Geometry: final body of the model. Coordinates: model frame, mm. A direction names the side the tool comes from. Give positions to 0.01 mm unless a question says otherwise; leave off trailing zeros. Write each loop counter-clockwise with the first axis right and the second up, starting at its lowest first coordinate (ties: lowest second). Pieces come first, ordered by that corner, then holes. Notation, with made-up numbers: (81.25, 5.25) -> (98.25, 5.25) arc R27 ccw to (98.25, 39.25) -> close; hole circle Ø11 at (-36, 45.25). An arc over 180 degrees is marked (long way). Answer in a Markdown table with one row per item. Add a question column.
from build123d import *

# Parameters (mm, degrees)
F1_DEPTH = 63.5
F2_DEPTH = 7.9375
F0_W     = 25.4
F0_H     = 19.05
F3_DEPTH = 25.4


with BuildPart() as f1:
    # F0 (on Front) → F1 (new body, symmetric)
    with BuildSketch(Plane.XZ):
        Polygon((22.225, 9.525), (-41.275, 9.525), (-41.275, -9.525), (41.275, -9.525), (41.275, 9.525), align=None)
    extrude(amount=F1_DEPTH, both=True)

    # F0 (on Front) → F2 (join, symmetric)
    with BuildSketch(Plane.XZ):
        with BuildLine():
            add(Edge.make_bspline(
                [(-41.275, 9.525), (-36.750946, 41.332115), (12.617621, 58.127224), (52.07476, 61.55447)],
                knots=[0, 0, 0, 0, 106.867946, 106.867946, 106.867946, 106.867946], degree=3))
            Line((-41.275, 9.525), (22.225, 9.525))
            Line((22.225, 9.525), (22.225, 27.0002))
            ThreePointArc((22.225, 27.0002), (30.72077, 49.831132), (52.07476, 61.55447))
        make_face()
    extrude(amount=F2_DEPTH, both=True)

    # F0 (on Front) → F3 (join, symmetric)
    with BuildSketch(Plane.XZ):
        with BuildLine():
            Line((22.225, 27.0002), (22.225, 9.525))
            Line((22.225, 9.525), (41.275, 9.525))
            Line((41.275, 9.525), (41.275, 27.0002))
            ThreePointArc((41.275, 27.0002), (45.92468, 38.22552), (57.15, 42.8752))
            Line((57.15, 42.8752), (73.83506, 42.8752))
            Line((73.83506, 42.8752), (73.83506, 61.9252))
            Line((73.83506, 61.9252), (57.15, 61.9252))
            add(Edge.make_bspline(
                [(52.07476, 61.55447), (53.786654, 61.703165), (55.479892, 61.826697), (57.15, 61.9252)],
                knots=[106.867946, 106.867946, 106.867946, 106.867946, 111.504536, 111.504536, 111.504536, 111.504536], degree=3))
            ThreePointArc((52.07476, 61.55447), (30.72077, 49.831132), (22.225, 27.0002))
        make_face()
        with Locations((86.53506, 52.4002)):
            Rectangle(F0_W, F0_H)
    extrude(amount=F3_DEPTH, both=True)

    # F0 (on Front) → F4 (revolve)
    with BuildSketch(Plane.XZ):
        Polygon((99.23506, 66.675), (99.23506, 61.9252), (99.23506, 42.8752), (99.23506, 38.1), (124.63506, 38.1), (124.63506, 66.675), align=None)
    revolve(axis=Axis((99.23506, 0, 52.3875), (0, 0, 1)))


solid = f1.part
Q1. Line query: probe 1 along Z at (x, y) = (-2, 17) (3 decimals); probe 2 along Z at (x, y) = (97.5, -12) (3 decimals); probe 3 along Y at (x, z) = (11, 20). Output: solid intervals per line, ascending. Write a range as from..to.
Q2. Section A-A on y = -37. Return loops of the section in (x, z) (3 decimals), and give its area (3 significant figures).
Q3. Access query for faces 4 (the flat face through (41.275, -1, 4)), 5 (the flat face through (52, -25.4, 48)), 6 (the flat face through (52, 25.4, 48)), 7 (the flat face through (22.225, -17, 18)), 8 (the cylindrical face through (30.95, 16.547, 50.094)). Directions: +Z, -Z, +X, -X, +Y, -Y. A direction counts if a zero-diameter tool reaches every point of the face in a straight line with its end or side. Return the directions, or none.
Q4. Pull-direction query (X, two-part tool) for faces 1 (the cylindrical face through (45.8, -0.4, 38.1)), 2 (the cylindrical face through (30.95, -16.791, 50.094)), 3 (the flat face through (-4, -7.938, 30)); classes: +X half, -X half, draft (parallel to the pull), parting line (faces both ways), or undercut.
Q5. Section B-B on z = -1.5. Return loops of the section in (x, y) (3 decimals), and give its area (3 significant figures).
Q6. Contact query for flat-ended pins moving along their axis: pin 1 Ø5 at (y, z) = (-19, 21) entering from -X (3 decimals); pin 2 Ø10 at (y, z) = (-3, 12) entering from +X (3 decimals); pin 3 Ø15.5 at (x, z) = (-13.5, 44.5) entering from -Y. Output: stop coordinate, or through.
Checks:
| question | item | result |
|---|---|---|
| 1 | probe 1 | -9.525..9.525 |
| 1 | probe 2 | 38.1..66.675 |
| 1 | probe 3 | -7.94..7.94 |
| 2 | outline | (-41.275, -9.525) -> (41.275, -9.525) -> (41.275, 9.525) -> (-41.275, 9.525) -> close |
| 2 | area | 1,570 mm^2 |
| 3 | face 4 | -Z, +X, +Y, -Y |
| 3 | face 5 | +Z, +X, -X, -Y |
| 3 | face 6 | +Z, +X, -X, +Y |
| 3 | face 7 | +Z, -X, -Y |
| 3 | face 8 | +Z, -X, +Y |
| 4 | face 1 | undercut |
| 4 | face 2 | -X half |
| 4 | face 3 | draft |
| 5 | outline | (-41.275, -63.5) -> (41.275, -63.5) -> (41.275, 63.5) -> (-41.275, 63.5) -> close |
| 5 | area | 10,500 mm^2 |
| 6 | pin 1 | x = 22.225 |
| 6 | pin 2 | x = 41.275 |
| 6 | pin 3 | y = -7.94 |
